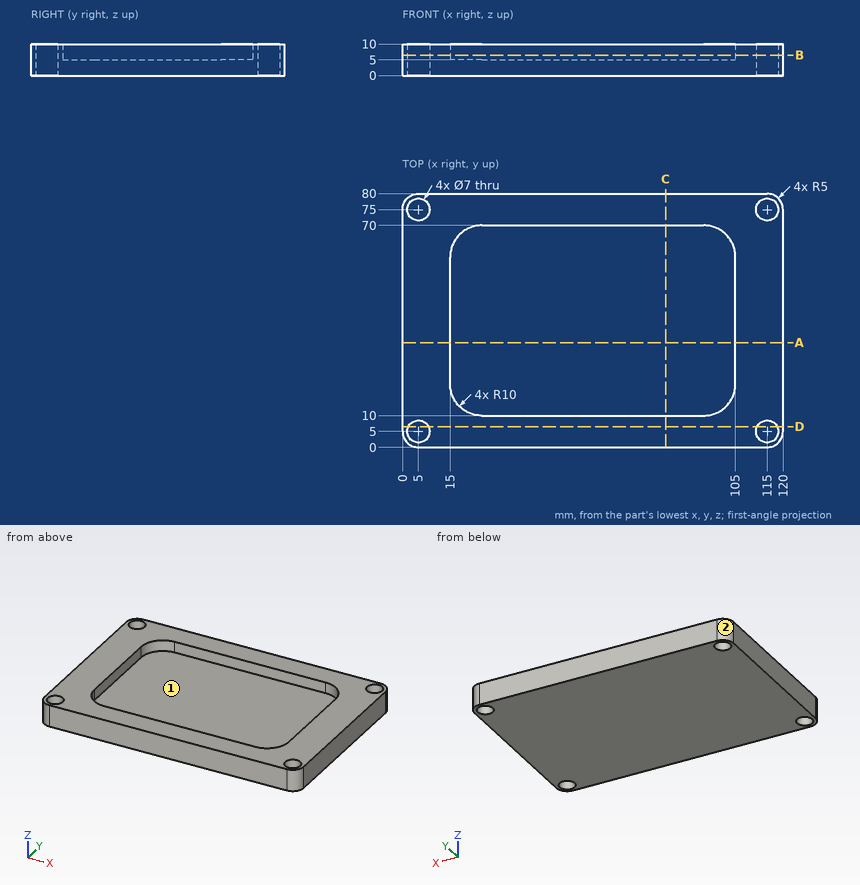
The drawing under review shows one solid part. Ordinate dimensions are in mm from its lowest x, y, z. A direction names the side the tool comes from. Coordinates: 2 decimals unless noted, no trailing zeros. Order: outer loops, then holes, each group sorted by start corner. A loop starts at its lowest first (then second) coordinate and runs counter-clockwise, first axis right, second up. Notation, with made-up numbers: (88.25, 59.25) -> (125.25, 59.25) arc R25 ccw to (125.25, 87.25) -> close; hole circle Ø11 at (53.5, 4). An arc over 180 degrees is marked (long way). Return JSON: item names as keys, results as strings.
1. For line 1 (Y direction, x = 5, z = 4.75); line 2 (Y direction, x = 50, z = 5.5); line 3 (X direction, y = 59, z = 5.5), list the stretches that pass through material, from the lowest coordinate up. Write a range as from..to.
Answer block:
{"line 1": "0..1.5, 8.5..71.5, 78.5..80", "line 2": "0..10, 70..80", "line 3": "0..15, 105..120"}
2. We need section B-B on z = 6.5. Write out the cut boundary in (x, y), and give its area (3 significant figures).
Answer block:
{"outline": "(0, 5) arc R5 ccw to (5, 0) -> (115, 0) arc R5 ccw to (120, 5) -> (120, 75) arc R5 ccw to (115, 80) -> (5, 80) arc R5 ccw to (0, 75) -> close; hole circle Ø7 at (5, 5); hole circle Ø7 at (5, 75); hole (15, 20) arc R10 ccw to (25, 10) -> (95, 10) arc R10 ccw to (105, 20) -> (105, 60) arc R10 ccw to (95, 70) -> (25, 70) arc R10 ccw to (15, 60) -> close; hole circle Ø7 at (115, 5); hole circle Ø7 at (115, 75)", "area": "4,110 mm²"}
3. We need section C-C on x = 83. Write out the cut boundary in (y, z), and give its area (3 significant figures).
Answer block:
{"outline": "(0, 0) -> (80, 0) -> (80, 10) -> (70, 10) -> (70, 5) -> (10, 5) -> (10, 10) -> (0, 10) -> close", "area": "500 mm²"}
4. Machinability: for the marked faces 1 and 2, which of the approach directions +Z, -Z, +X, -X, +Y, -Y give a long, thin tool a straight path to every point of the face, cutting with its end or side? Answer none if there is none.
Answer block:
{"face 1": "+Z", "face 2": "+Z, -Z, -X, +Y"}
5. We need section A-A on y = 33. Write out the cut boundary in (x, z).
Answer block:
{"outline": "(0, 0) -> (120, 0) -> (120, 10) -> (105, 10) -> (105, 5) -> (15, 5) -> (15, 10) -> (0, 10) -> close"}
6. For pin 1 Ø12 at (x, y) = (69.5, 44.5) entering from +Z, flat-tipped, find the tip position at first contact; note if it passes through.
Answer block:
{"pin 1": "z = 5"}
7. We need section D-D on y = 6.5. Write out the cut boundary in (x, z), and give its area (3 significant figures).
Answer block:
{"outline": "(0, 0) -> (1.84, 0) -> (1.84, 10) -> (0, 10) -> close; (8.16, 0) -> (111.84, 0) -> (111.84, 10) -> (8.16, 10) -> close; (118.16, 0) -> (120, 0) -> (120, 10) -> (118.16, 10) -> close", "area": "1,070 mm²"}
